The drawing under review shows one solid part. Ordinate dimensions are in mm from its lowest x, y, z. A direction names the side the tool comes from. Round coordinates to 2 decimals unless told otherwise and drop trailing zeros. Order: outer loops, then holes, each group sorted by start corner. A loop starts at its lowest first (then second) coordinate and runs counter-clockwise, first axis right, second up. Notation, with made-up numbers: M 26.25,82 L 46.25,82 A32 ccw 46.25,114 Z; hole C -4,-34 d2. An arc over 180 degrees is marked long. Use a Markdown table: item, result.
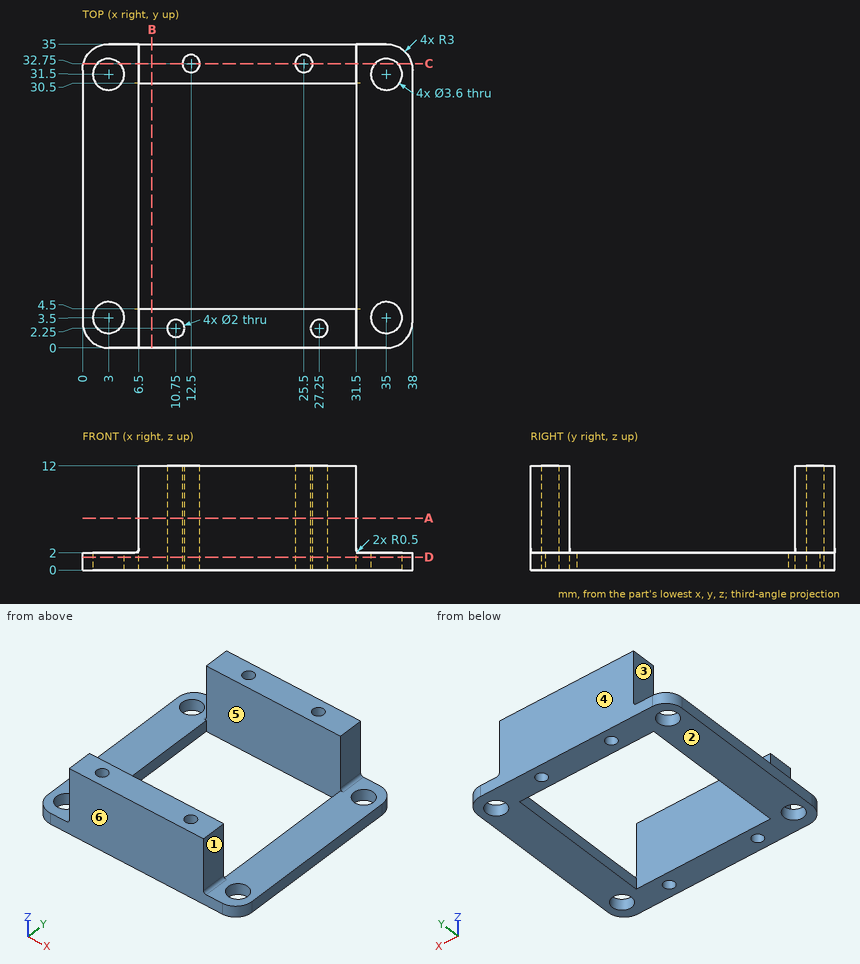
Q1. Clearance check with flat-ended pins moving along their axes: pin 1 (3.5 mm diameter, centred on y = 3, z = 8.5, fed in from +X); pin 2 (3 mm diameter, centred on x = 3, y = 31.5, fed in from -Z); pin 3 (3.5 mm diameter, centred on x = 21, z = 5, fed in from -Y); pin 4 (4.5 mm diameter, centred on x = 35, y = 31.5, fed in from +Z). State where each tip first meets the part, or that it passes through.
Determined:
| item | result |
|---|---|
| pin 1 | stops at x = 31.5 |
| pin 2 | passes through |
| pin 3 | stops at y = 0 |
| pin 4 | stops at z = 2 |
Q2. Machinability: for the marked faces 1, 2 and 3, which of the approach directions +Z, -Z, +X, -X, +Y, -Y give a long, thin tool a straight path to every point of the face, cutting with its end or side? Answer none if there is none.
Determined:
| item | result |
|---|---|
| face 1 | +Z, +X, +Y, -Y |
| face 2 | -Z, +X, -X, +Y, -Y |
| face 3 | +Z, -X, +Y, -Y |
Q3. Add section B-B (x = 8). Write out the cut boundary in (y, z).
Determined:
| item | result |
|---|---|
| outline | M 0,0 L 4.5,0 L 4.5,12 L 0,12 Z; M 30.5,0 L 35,0 L 35,12 L 30.5,12 Z |
Q4. Add section C-C (y = 32.75). Write out the cut boundary in (x, z), then the cut area to 3 significant figures.
Determined:
| item | result |
|---|---|
| outline | M 0.1,0 L 1.7,0 L 1.7,2 L 0.1,2 Z; M 4.3,0 L 11.5,0 L 11.5,12 L 6.5,12 L 6.5,2.5 A0.5 cw 6,2 L 4.3,2 Z; M 13.5,0 L 24.5,0 L 24.5,12 L 13.5,12 Z; M 26.5,0 L 33.7,0 L 33.7,2 L 32,2 A0.5 cw 31.5,2.5 L 31.5,12 L 26.5,12 Z; M 36.3,0 L 37.9,0 L 37.9,2 L 36.3,2 Z |
| area | 267 mm^2 |
Q5. Add section D-D (z = 1.5). Give the number of separate pieces and of enclosed holes in the cut face, then the cut area to 3 significant figures.
Determined:
| item | result |
|---|---|
| separate pieces | 1 |
| enclosed holes | 9 |
| area | 619 mm^2 |
Q6. Wall thickness on line 1 along Y through (x, z) = (35, 0.55); line 2 along X through (y, z) = (32.5, 6.5); line 3 along Y through (x, z) = (23, 11.25): over which ranges is each line inside the solid? List them lowest first. Write a range as [from, to].
Determined:
| item | result |
|---|---|
| line 1 | y = [0, 1.7], [5.3, 29.7], [33.3, 35] |
| line 2 | x = [6.5, 11.53], [13.47, 24.53], [26.47, 31.5] |
| line 3 | y = [0, 4.5], [30.5, 35] |
Q7. Draft analysis for pull direction Y (two halves, no side actions). For the marked faces 4, 5 and 6, state which applies: pulls with the +Y half, pulls with the -Y half, needs draft (parallel to the pull), parting line crosses it, or undercut.
Determined:
| item | result |
|---|---|
| face 4 | pulls with the +Y half |
| face 5 | undercut |
| face 6 | pulls with the -Y half |
Q8. Add section A-A (z = 6). Write out the cut boundary in (x, y).
Determined:
| item | result |
|---|---|
| outline | M 6.5,0 L 31.5,0 L 31.5,4.5 L 6.5,4.5 Z; M 6.5,30.5 L 31.5,30.5 L 31.5,35 L 6.5,35 Z; hole C 10.75,2.25 d2; hole C 12.5,32.75 d2; hole C 25.5,32.75 d2; hole C 27.25,2.25 d2 |
